Geometry check sheet. Reference: the model listing, model coordinates, mm. Face numbers are marked on the shaded views. Round coordinates to 2 decimals unless told otherwise and drop trailing zeros. Order: outer loops, then holes, each group sorted by start corner. A loop starts at its lowest first (then second) coordinate and runs counter-clockwise, first axis right, second up. Notation, with made-up numbers: (14.25, -20.5) -> (18.25, -20.5) arc R30 cw to (18.25, 13.5) -> close; hole circle Ø8 at (-1, 1). An arc over 180 degrees is marked (long way). Answer as a JSON object with one key per item and string values. Group by question number.
from build123d import *

# Parameters (mm, degrees)
F0_R     = 4
F1_DEPTH = 8


with BuildPart() as f1:
    # F0 (on Top) → F1 (new body)
    with BuildSketch(Plane.XY):
        with BuildLine():
            Line((0, 85.948586), (0, 10))
            ThreePointArc((0, 10), (2.928932, 2.928932), (10, 0))
            ThreePointArc((10, 0), (17.071068, 2.928932), (20, 10))
            Line((20, 10), (20, 85.948586))
            Line((20, 85.948586), (10, 120))
            Line((10, 120), (0, 85.948586))
        make_face()
        with Locations((10, 15)):
            Circle(F0_R, mode=Mode.SUBTRACT)
    extrude(amount=F1_DEPTH)


solid = f1.part
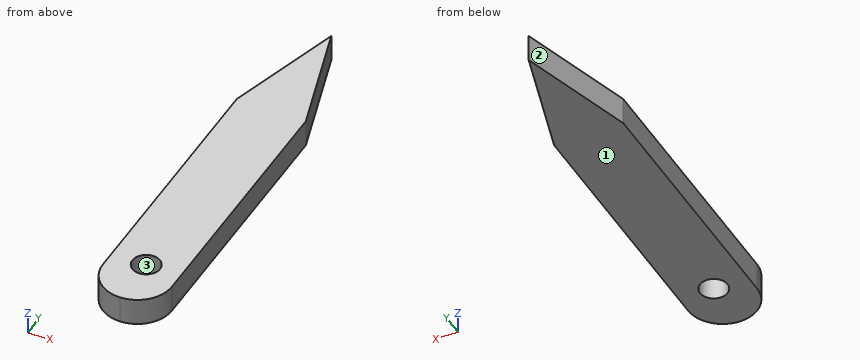
Item 1: Thickness scan on L1, parallel to X at y = 12, z = 4. Record the ranges inside material, lowest first.
Item 2: Mould release check, pull along X, two halves, no side actions. Record for the marked faces 1, 2 and 3: pulls with the +X half, pulls with the -X half, needs draft (parallel to the pull), parting line crosses it, or undercut.
Item 3: Sectioned sample at A-A, the plane y = 15. Enter the section's corners in (x, z).
Item 4: Sectioned sample at B-B, the plane x = 11.5. Enter the section's corners in (y, z), then the cut area to 3 significant figures.
Item 5: Sectioned sample at D-D, the plane y = 94. Enter the section's corners in (x, z).
Item 6: Sectioned sample at C-C, the plane z = 5.25. Enter the section's corners in (x, y), then the cut area to 3 significant figures.
Result:
{
 "1": {"L1": "x = 0 to 7.35, 12.65 to 20"},
 "2": {"face 1": "needs draft", "face 2": "pulls with the -X half", "face 3": "undercut"},
 "3": {"outline": "(0, 0) -> (6, 0) -> (6, 8) -> (0, 8) -> close; (14, 0) -> (20, 0) -> (20, 8) -> (14, 8) -> close"},
 "4": {"outline": "(0.11, 0) -> (11.29, 0) -> (11.29, 8) -> (0.11, 8) -> close; (18.71, 0) -> (114.89, 0) -> (114.89, 8) -> (18.71, 8) -> close", "area": "859 mm2"},
 "5": {"outline": "(2.36, 0) -> (17.64, 0) -> (17.64, 8) -> (2.36, 8) -> close"},
 "6": {"outline": "(0, 10) arc R10 ccw to (10, 0) arc R10 ccw to (20, 10) -> (20, 85.95) -> (10, 120) -> (0, 85.95) -> close; hole circle Ø8 at (10, 15)", "area": "1,970 mm2"}
}
